from build123d import *

# Parameters (mm, degrees)
SKETCH2_W           = 13
SKETCH2_H           = 20
BOSS_EXTRUDE1_DEPTH = 6
BOSS_EXTRUDE2_DEPTH = 2
BOSS_EXTRUDE3_START = 1
SKETCH3_W           = 13
SKETCH3_H           = 20
SKETCH3_R           = 3.2
BOSS_EXTRUDE3_DEPTH = 1
BOSS_EXTRUDE4_DEPTH = 4
CUT_EXTRUDE1_START  = -6
CUT_EXTRUDE1_DEPTH  = 6
BOSS_EXTRUDE5_DEPTH = 2
SKETCH8_R           = 3.2
SKETCH8_R_2         = 3.1
BOSS_EXTRUDE6_DEPTH = 7
SKETCH9_W           = 1.7
SKETCH9_H           = 15.38
CUT_EXTRUDE2_DEPTH  = 4


# Read off the part's stored shape, not the designer's step: Cut-Extrude1
with BuildPart() as part:
    # Sketch2 → Boss-Extrude1 (new body)
    with BuildSketch(Plane.XY):
        Rectangle(SKETCH2_W, SKETCH2_H)
        with BuildLine():
            Line((1.3, -9.04), (1.3, -2.924038303))
            ThreePointArc((1.3, -2.924038303), (-3.2, 0), (1.3, 2.924038303))
            Line((1.3, 2.924038303), (1.3, 9.04))
            Line((1.3, 9.04), (5.7, 9.04))
            Line((5.7, 9.04), (5.7, -9.04))
            Line((5.7, -9.04), (1.3, -9.04))
        make_face(mode=Mode.SUBTRACT)
    extrude(amount=BOSS_EXTRUDE1_DEPTH)

    # Sketch2<3> → Boss-Extrude2 (add)
    with BuildSketch(Plane.XY):
        with BuildLine():
            Line((4.2, 7.54), (4.2, -7.54))
            Line((4.2, -7.54), (2.8, -7.54))
            Line((2.8, -7.54), (2.8, -1.549193338))
            ThreePointArc((2.8, -1.549193338), (2.162186317, -2.359014695), (1.3, -2.924038303))
            Line((1.3, -2.924038303), (1.3, -9.04))
            Line((1.3, -9.04), (5.7, -9.04))
            Line((5.7, -9.04), (5.7, 9.04))
            Line((5.7, 9.04), (1.3, 9.04))
            Line((1.3, 9.04), (1.3, 2.924038303))
            ThreePointArc((1.3, 2.924038303), (2.162186317, 2.359014695), (2.8, 1.549193338))
            Line((2.8, 1.549193338), (2.8, 7.54))
            Line((2.8, 7.54), (4.2, 7.54))
        make_face()
    extrude(amount=BOSS_EXTRUDE2_DEPTH)

    # Sketch3 → Boss-Extrude3 (add)
    with BuildSketch(Plane(origin=(0, 0, 0), x_dir=(-1, 0, 0), z_dir=(0, 0, -1)).offset(BOSS_EXTRUDE3_START)):
        Rectangle(SKETCH3_W, SKETCH3_H)
        Circle(SKETCH3_R, mode=Mode.SUBTRACT)
    extrude(amount=-BOSS_EXTRUDE3_DEPTH)

    # Sketch4 → Boss-Extrude4 (add)
    with BuildSketch(Plane.XY.offset(2)):
        with BuildLine():
            Line((2.8, 1.549193338), (2.8, 7.54))
            Line((2.8, 7.54), (4.2, 7.54))
            Line((4.2, 7.54), (4.2, -7.54))
            Line((4.2, -7.54), (2.8, -7.54))
            Line((2.8, -7.54), (2.8, -1.549193338))
            ThreePointArc((2.8, -1.549193338), (2.162186317, -2.359014695), (1.3, -2.924038303))
            Line((1.3, -2.924038303), (1.3, -9.04))
            Line((1.3, -9.04), (5.7, -9.04))
            Line((5.7, -9.04), (5.7, 9.04))
            Line((5.7, 9.04), (1.3, 9.04))
            Line((1.3, 9.04), (1.3, 2.924038303))
            ThreePointArc((1.3, 2.924038303), (2.162186317, 2.359014695), (2.8, 1.549193338))
        make_face()
    extrude(amount=BOSS_EXTRUDE4_DEPTH)

    # Cut-Extrude1 outline → Cut-Extrude1 (cut)
    with BuildSketch(Plane.XY.offset(6).offset(CUT_EXTRUDE1_START)):
        with BuildLine():
            Line((4.35, 7.69), (2.65, 7.69))
            Line((2.65, 7.69), (2.65, 1.793739111))
            ThreePointArc((2.65, 1.793739111), (2.727741861, 1.673148033), (2.8, 1.549193338))
            Line((2.8, 1.549193338), (2.8, 7.54))
            Line((2.8, 7.54), (4.2, 7.54))
            Line((4.2, 7.54), (4.2, -7.54))
            Line((4.2, -7.54), (2.8, -7.54))
            Line((2.8, -7.54), (2.8, -1.549193338))
            ThreePointArc((2.8, -1.549193338), (2.727741861, -1.673148033), (2.65, -1.793739111))
            Line((2.65, -1.793739111), (2.65, -7.69))
            Line((2.65, -7.69), (4.35, -7.69))
            Line((4.35, -7.69), (4.35, 7.69))
        make_face()
    extrude(amount=CUT_EXTRUDE1_DEPTH, mode=Mode.SUBTRACT)

    # Sketch7 → Boss-Extrude5 (add)
    with BuildSketch(Plane.XY):
        with BuildLine():
            Line((2.65, 7.69), (2.65, 1.793739111))
            ThreePointArc((2.65, 1.793739111), (3.2, 0), (2.65, -1.793739111))
            Line((2.65, -1.793739111), (2.65, -7.69))
            Line((2.65, -7.69), (4.35, -7.69))
            Line((4.35, -7.69), (4.35, 7.69))
            Line((4.35, 7.69), (2.65, 7.69))
        make_face()
    extrude(amount=BOSS_EXTRUDE5_DEPTH)

    # Sketch8 → Boss-Extrude6 (add)
    with BuildSketch(Plane(origin=(0, 0, -1), x_dir=(-1, 0, 0), z_dir=(0, 0, -1))):
        Circle(SKETCH8_R)
        Circle(SKETCH8_R_2, mode=Mode.SUBTRACT)
    extrude(amount=-BOSS_EXTRUDE6_DEPTH)

    # Sketch9 → Cut-Extrude2 (cut)
    with BuildSketch(Plane.XY.offset(6)):
        with Locations((3.5, 0)):
            Rectangle(SKETCH9_W, SKETCH9_H)
    extrude(amount=-CUT_EXTRUDE2_DEPTH, mode=Mode.SUBTRACT)


solid = part.part
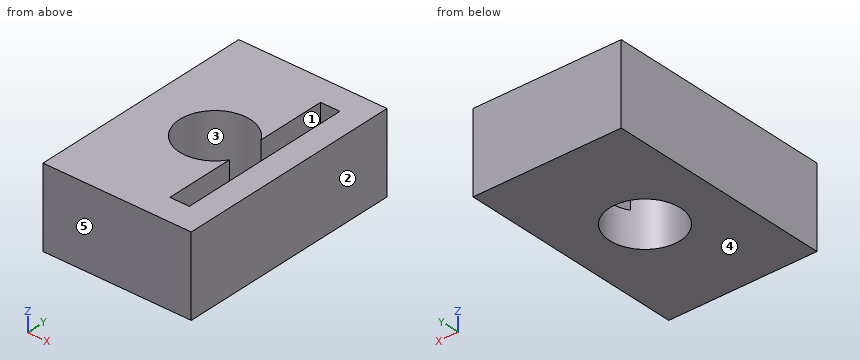
Geometry check sheet. Reference: the model listing, model coordinates, mm. Face numbers are marked on the shaded views. A direction names the side the tool comes from. Round coordinates to 2 decimals unless told otherwise and drop trailing zeros. Order: outer loops, then holes, each group sorted by start corner. A loop starts at its lowest first (then second) coordinate and runs counter-clockwise, first axis right, second up. Notation, with made-up numbers: M -19,68 L 39,68 A23 cw 39,106 Z; hole C 81.25,55.25 d10. An arc over 180 degrees is marked long. Write each question's results on one line, items separated by ' | '. Start each with the question number.
1. Set-up check for the marked faces 1 and 2: record each of +Z, -Z, +X, -X, +Y, -Y from which the full face is reachable in a straight line by a thin tool's end or side.
2. Draft check along Y on the marked faces 3, 4 and 5. Enter one of: pulls with the +Y half, pulls with the -Y half, needs draft (parallel to the pull), parting line crosses it, or undercut.
3. Cross-section at B-B on y = 0. Record the boundary of the cut face in (x, z).
4. Material ranges on L1, parallel to Y at x = 0, z = 4; L2, parallel to X at y = -4, z = 3.5; L3, parallel to X at y = 0, z = 1.5, recorded low to high. Write a range as from..to.
5. Cross-section at C-C on z = 5.25. Record the boundary of the cut face in (x, y).
6. Cross-section at D-D on y = -5. Record the boundary of the cut face in (x, z).
7. Cross-section at A-A on x = 0. Record the boundary of the cut face in (y, z), plus the area to 3 significant figures.
Resolved:
1) face 1: +Z | face 2: +Z, -Z, +X, +Y, -Y
2) face 3: undercut | face 4: needs draft | face 5: pulls with the -Y half
3) outline: M -6.5,-1 L -3.1,-1 L -3.1,6 L -6.5,6 Z; M 3.1,-1 L 6.5,-1 L 6.5,6 L 4.35,6 L 4.35,2 L 3.1,2 Z
4) L1: -10..-3.1, 3.1..10 | L2: -6.5..2.65, 4.35..6.5 | L3: -6.5..-3.1, 3.1..6.5
5) outline: M -6.5,-10 L 6.5,-10 L 6.5,10 L -6.5,10 Z; hole M 2.65,-7.69 L 4.35,-7.69 L 4.35,7.69 L 2.65,7.69 L 2.65,1.61 A3.1 ccw long 2.65,-1.61 Z
6) outline: M -6.5,-1 L 6.5,-1 L 6.5,6 L 4.35,6 L 4.35,2 L 2.65,2 L 2.65,6 L -6.5,6 Z
7) outline: M -10,-1 L -3.1,-1 L -3.1,6 L -10,6 Z; M 3.1,-1 L 10,-1 L 10,6 L 3.1,6 Z | area: 96.6 mm2
